Build history of the part. All positions in model axes, mm. Round coordinates to 2 decimals unless told otherwise and drop trailing zeros. Write each loop counter-clockwise with the first axis right and the second up, starting at its lowest first coordinate (ties: lowest second). Pieces come first, ordered by that corner, then holes. Notation, with made-up numbers: (-21, -15) - (18, -15) arc R19 cw to (18, 6) - close; hole circle Ø8 at (-19, 36). An arc over 180 degrees is marked (long way). Answer as a JSON object with one key per item and string values. Group by question number.
Item 1: Probe line 1 (Y direction, x = -0.85, z = -76.2); line 2 (Z direction, x = -0.1, y = -7); line 3 (Y direction, x = -1.1, z = 70). List the from-to ranges inside material, lowest first. Write a range as from..to.
Item 2: Slice it at D-D, the plane x = -0.85. Give the number of separate pieces and of enclosed holes in the cut face, then the cut area to 3 significant figures.
Item 3: Slice it at C-C, the plane z = 76.2. List the corners of the cut face in (x, y).
Item 4: Slice it at A-A, the plane z = 25.4. List the corners of the cut face in (x, y), then the cut area to 3 significant figures.
Item 5: Slice it at B-B, the plane z = -70.5. List the corners of the cut face in (x, y), then the cut area to 3 significant figures.
Item 6: Flat gauge pin, fed straight in: pin 1 (5.5 mm diameter, centred on y = -33.5, z = 25.4, fed in from -X). Where does the tip first touch, or does it go through?
from build123d import *

# Parameters (mm, degrees)
SKETCH1_W               = 228.6
SKETCH1_H               = 127
BASE_FLANGE1_DEPTH      = 1.1938
CUT_EXTRUDE1_REACH      = 132.76
SKETCH6_R               = 3.571875
SKETCH6_W               = 22.89175
SKETCH6_H               = 41.94175
LPATTERN1_COUNT         = 4
LPATTERN1_PITCH         = 50.8
CUT_EXTRUDE2_REACH      = 132.76
SKETCH7_R               = 3.571875
MIRROR2_COPY_1_REACH    = 132.76
MIRROR2_COPY_1_SKETCH_R = 3.571875
FILLET1_R               = 6.35
FILLET2_R               = 0.396875


# Sheet-metal steps are written as plain solids
with BuildPart() as part:
    # Sketch1 → Base-Flange1 (new body)
    with BuildSketch(Plane(origin=(0, 0, 0), x_dir=(0, 0, -1), z_dir=(1, 0, 0))):
        Rectangle(SKETCH1_W, SKETCH1_H)
    extrude(amount=-BASE_FLANGE1_DEPTH)

    # Sketch6 → Cut-Extrude1 (cut, up to next)
    with BuildSketch(Plane(origin=(0, 0, 0), x_dir=(0, 0, -1), z_dir=(1, 0, 0)), mode=Mode.PRIVATE) as cut_extrude1_sk1:
        with Locations((-76.2, 33.5026)):
            Circle(SKETCH6_R)
    cut_extrude1_tool1 = extrude(cut_extrude1_sk1.sketch, amount=-CUT_EXTRUDE1_REACH, mode=Mode.PRIVATE) & part.part
    # Sketch6 → Cut-Extrude1 (cut, up to next)
    with BuildSketch(Plane(origin=(0, 0, 0), x_dir=(0, 0, -1), z_dir=(1, 0, 0)), mode=Mode.PRIVATE) as cut_extrude1_sk2:
        with Locations((-76.2, -33.5026)):
            Circle(SKETCH6_R)
    cut_extrude1_tool2 = extrude(cut_extrude1_sk2.sketch, amount=-CUT_EXTRUDE1_REACH, mode=Mode.PRIVATE) & part.part
    # Sketch6 → Cut-Extrude1 (cut, up to next)
    with BuildSketch(Plane(origin=(0, 0, 0), x_dir=(0, 0, -1), z_dir=(1, 0, 0)), mode=Mode.PRIVATE) as cut_extrude1_sk3:
        with Locations((-76.2, 0)):
            Rectangle(SKETCH6_W, SKETCH6_H)
    cut_extrude1_tool3 = extrude(cut_extrude1_sk3.sketch, amount=-CUT_EXTRUDE1_REACH, mode=Mode.PRIVATE) & part.part
    cut_extrude1_1 = cut_extrude1_tool1.solids().sort_by_distance((0, 33.5026, 76.2))[0]
    add(cut_extrude1_1, mode=Mode.SUBTRACT)
    cut_extrude1_2 = cut_extrude1_tool2.solids().sort_by_distance((0, -33.5026, 76.2))[0]
    add(cut_extrude1_2, mode=Mode.SUBTRACT)
    cut_extrude1_3 = cut_extrude1_tool3.solids().sort_by_distance((0, 0, 76.2))[0]
    add(cut_extrude1_3, mode=Mode.SUBTRACT)
    cut_extrude1 = cut_extrude1_1 + cut_extrude1_2 + cut_extrude1_3  # Cut-Extrude1 as one shape, for the pattern or mirror that repeats it

    # LPattern1: Cut-Extrude1 ×4
    with Locations(*[(0, 0, -i * LPATTERN1_PITCH) for i in range(1, LPATTERN1_COUNT)]):
        add(cut_extrude1, mode=Mode.SUBTRACT)

    # Sketch7 → Cut-Extrude2 (cut, up to next)
    with BuildSketch(Plane(origin=(0, 0, 0), x_dir=(0, 0, -1), z_dir=(1, 0, 0)), mode=Mode.PRIVATE) as cut_extrude2_sk1:
        with Locations((-76.2, 53.975)):
            Circle(SKETCH7_R)
    cut_extrude2_tool1 = extrude(cut_extrude2_sk1.sketch, amount=-CUT_EXTRUDE2_REACH, mode=Mode.PRIVATE) & part.part
    cut_extrude2 = cut_extrude2_tool1.solids().sort_by_distance((0, 53.975, 76.2))[0]
    add(cut_extrude2, mode=Mode.SUBTRACT)

    # Mirror1: Cut-Extrude2 across plane
    add(cut_extrude2.mirror(Plane.XY), mode=Mode.SUBTRACT)

    # Mirror2: Cut-Extrude2 across plane
    add(cut_extrude2.mirror(Plane.ZX), mode=Mode.SUBTRACT)

    # Mirror2 copy 1 sketch → Mirror2 copy 1 (cut, up to next)
    with BuildSketch(Plane(origin=(0, 0, 0), x_dir=(0, 0, 1), z_dir=(1, 0, 0)), mode=Mode.PRIVATE) as mirror2_copy_1_sk1:
        with Locations((-76.2, 53.975)):
            Circle(MIRROR2_COPY_1_SKETCH_R)
    mirror2_copy_1_tool1 = extrude(mirror2_copy_1_sk1.sketch, amount=-MIRROR2_COPY_1_REACH, mode=Mode.PRIVATE) & part.part
    add(mirror2_copy_1_tool1.solids().sort_by_distance((0, -53.975, -76.2))[0], mode=Mode.SUBTRACT)

    # Fillet1
    fillet1_edges = [part.edges().sort_by_distance(p)[0] for p in [
        (-0.5969, 63.5, 114.3),
        (-0.5969, 63.5, -114.3),
        (-0.5969, -63.5, -114.3),
        (-0.5969, -63.5, 114.3),
    ]]
    fillet(fillet1_edges, radius=FILLET1_R)

    # Fillet2
    fillet2_edges = [part.edges().sort_by_distance(p)[0] for p in [
        (-0.5969, 20.970875, 64.754125),
        (-0.5969, -20.970875, 64.754125),
        (-0.5969, -20.970875, 87.645875),
        (-0.5969, 20.970875, 87.645875),
        (-0.5969, 20.970875, 13.954125),
        (-0.5969, -20.970875, 13.954125),
        (-0.5969, -20.970875, 36.845875),
        (-0.5969, 20.970875, 36.845875),
        (-0.5969, -20.970875, -36.845875),
        (-0.5969, 20.970875, -36.845875),
        (-0.5969, -20.970875, -13.954125),
        (-0.5969, 20.970875, -13.954125),
        (-0.5969, -20.970875, -87.645875),
        (-0.5969, 20.970875, -87.645875),
        (-0.5969, -20.970875, -64.754125),
        (-0.5969, 20.970875, -64.754125),
    ]]
    fillet(fillet2_edges, radius=FILLET2_R)


solid = part.part
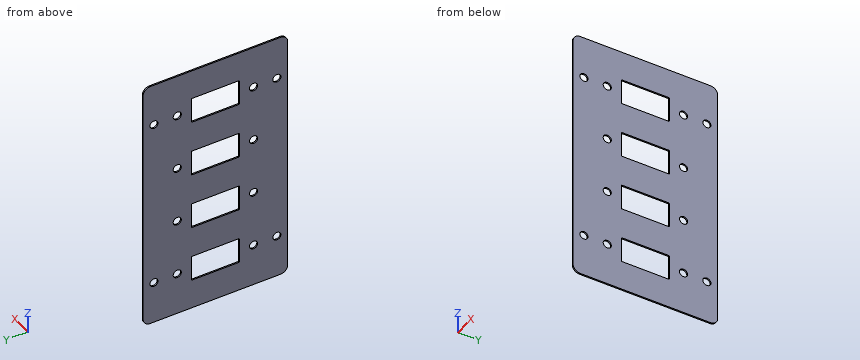
Geometry says:
{
 "1": {"line 1": "y = -63.5..-57.55, -50.4..-37.07, -29.93..-20.97, 20.97..29.93, 37.07..50.4, 57.55..63.5", "line 2": "z = -114.3..-87.65, -64.75..-36.85, -13.95..13.95, 36.85..64.75, 87.65..114.3", "line 3": "y = -63.5..-20.97, 20.97..63.5"},
 "2": {"separate pieces": "1", "enclosed holes": "16", "area": "24,700 mm^2"},
 "3": {"outline": "(-1.19, -63.5) - (0, -63.5) - (0, -57.55) - (-1.19, -57.55) - close; (-1.19, -50.4) - (0, -50.4) - (0, -37.07) - (-1.19, -37.07) - close; (-1.19, -29.93) - (0, -29.93) - (0, -20.97) - (-1.19, -20.97) - close; (-1.19, 20.97) - (0, 20.97) - (0, 29.93) - (-1.19, 29.93) - close; (-1.19, 37.07) - (0, 37.07) - (0, 50.4) - (-1.19, 50.4) - close; (-1.19, 57.55) - (0, 57.55) - (0, 63.5) - (-1.19, 63.5) - close"},
 "4": {"outline": "(-1.19, -63.5) - (0, -63.5) - (0, -37.07) - (-1.19, -37.07) - close; (-1.19, -29.93) - (0, -29.93) - (0, -20.97) - (-1.19, -20.97) - close; (-1.19, 20.97) - (0, 20.97) - (0, 29.93) - (-1.19, 29.93) - close; (-1.19, 37.07) - (0, 37.07) - (0, 63.5) - (-1.19, 63.5) - close", "area": "84.5 mm^2"},
 "5": {"outline": "(-1.19, -63.5) - (0, -63.5) - (0, -20.97) - (-1.19, -20.97) - close; (-1.19, 20.97) - (0, 20.97) - (0, 63.5) - (-1.19, 63.5) - close", "area": "102 mm^2"},
 "6": {"pin 1": "passes through"}
}
